Can you work these out from the model? Positions are in its coordinate system, mm. Round coordinates to 2 decimals unless told otherwise and drop trailing zeros. Loops run counter-clockwise (first coordinate to the right, second up) from the corner with the lowest first, then second, coordinate; pieces in that order, holes last. Notation, with made-up numbers: (18.25, 25) -> (75.25, 25) arc R25 ccw to (75.25, 41) -> close; hole circle Ø1 at (-34.5, 38). An arc over 180 degrees is marked (long way). Answer as a JSON object with one key per item and string values.
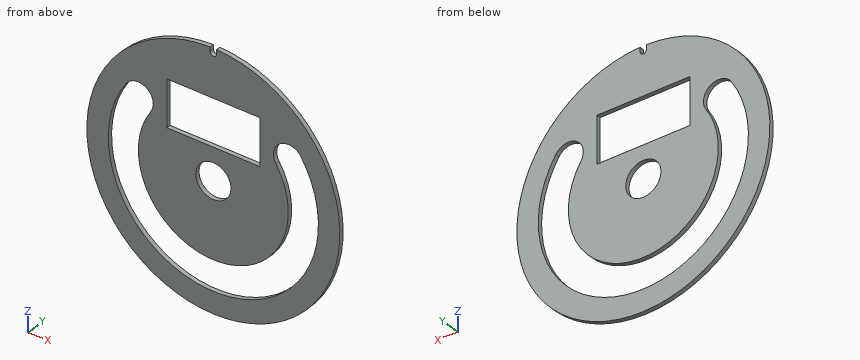
```python
from build123d import *

# Parameters (mm, degrees)
SKETCH_1_R      = 4.1
SKETCH_1_W      = 21.7
SKETCH_1_H      = 10.85
EXTRUDE_1_DEPTH = 1


with BuildPart() as part:
    # Эскиз1 → Бобышка-Вытянуть1 (new body)
    with BuildSketch(Plane(origin=(0, 0, 0), x_dir=(1, 0, 0), z_dir=(0, 1, 0))):
        with BuildLine():
            Line((0.75, -28.503654365), (0.75, -29.46545647))
            ThreePointArc((0.75, -29.46545647), (0, 29.475), (-0.75, -29.46545647))
            Line((-0.75, -29.46545647), (-0.75, -28.503654365))
            ThreePointArc((-0.75, -28.503654365), (0, -27.732186207), (0.75, -28.503654365))
        make_face()
        Circle(SKETCH_1_R, mode=Mode.SUBTRACT)
        with Locations((0, -12.957484911)):
            Rectangle(SKETCH_1_W, SKETCH_1_H, mode=Mode.SUBTRACT)
        with BuildLine():
            ThreePointArc((20.420143027, -13.492345376), (0, 24.475), (-20.420143027, -13.492345376))
            ThreePointArc((-20.420143027, -13.492345376), (-15.570553266, -14.483041669), (-14.579856973, -9.633451908))
            ThreePointArc((-14.579856973, -9.633451908), (0, 17.475), (14.579856973, -9.633451908))
            ThreePointArc((14.579856973, -9.633451908), (15.570553266, -14.483041669), (20.420143027, -13.492345376))
        make_face(mode=Mode.SUBTRACT)
    extrude(amount=EXTRUDE_1_DEPTH)


solid = part.part
```
Q1. I want a section at D-D, the plane y = 0.7. Write out the boundary of the cut face in (x, z) (3 decimals).
Determined:
{"outline": "(-0.75, 28.504) -> (-0.75, 29.465) arc R29.475 ccw (long way) to (0.75, 29.465) -> (0.75, 28.504) arc R0.75 cw (long way) to start; hole (-20.42, 13.492) arc R24.475 ccw (long way) to (20.42, 13.492) arc R3.5 ccw to (14.58, 9.633) arc R17.475 cw (long way) to (-14.58, 9.633) arc R3.5 ccw to start; hole (-10.85, 7.532) -> (10.85, 7.532) -> (10.85, 18.382) -> (-10.85, 18.382) -> close; hole circle Ø8.2 at (0, 0)"}
Q2. I'm going to push flat-ended pins straight in: pin 1 (0.5 mm diameter, centred on x = 4, y = 0.5, fed in from +Z); pin 2 (0.5 mm diameter, centred on x = 2, y = 0.5, fed in from -Z); pin 3 (4 mm diameter, centred on x = 16.5, z = 9, fed in from -Y). Where does each tip first touch, or does it pass through?
Determined:
{"pin 1": "z = 29.24", "pin 2": "z = -29.42", "pin 3": "y = 0"}
Q3. I want a section at C-C, the plane z = -8. Write out the boundary of the cut face in (x, y), then the cut area to 3 significant figures.
Determined:
{"outline": "(-28.37, 0) -> (-23.13, 0) -> (-23.13, 1) -> (-28.37, 1) -> close; (-15.54, 0) -> (15.54, 0) -> (15.54, 1) -> (-15.54, 1) -> close; (23.13, 0) -> (28.37, 0) -> (28.37, 1) -> (23.13, 1) -> close", "area": "41.5 mm²"}
Q4. I want a section at B-B, the plane z = 0. Write out the boundary of the cut face in (x, y) (3 decimals), then the cut area to 4 significant figures.
Determined:
{"outline": "(-29.475, 0) -> (-24.475, 0) -> (-24.475, 1) -> (-29.475, 1) -> close; (-17.475, 0) -> (-4.1, 0) -> (-4.1, 1) -> (-17.475, 1) -> close; (4.1, 0) -> (17.475, 0) -> (17.475, 1) -> (4.1, 1) -> close; (24.475, 0) -> (29.475, 0) -> (29.475, 1) -> (24.475, 1) -> close", "area": "36.75 mm²"}
Q5. I want a section at A-A, the plane x = 0. Write out the boundary of the cut face in (y, z) (3 decimals), then the cut area to 3 significant figures.
Determined:
{"outline": "(0, -29.475) -> (1, -29.475) -> (1, -24.475) -> (0, -24.475) -> close; (0, -17.475) -> (1, -17.475) -> (1, -4.1) -> (0, -4.1) -> close; (0, 4.1) -> (1, 4.1) -> (1, 7.532) -> (0, 7.532) -> close; (0, 18.382) -> (1, 18.382) -> (1, 27.732) -> (0, 27.732) -> close", "area": "31.2 mm²"}
Q6. If I drill on L1, parallel to X at y = 0.65, z = 0 (3 decimals); L2, parallel to Z at x = -6.5, y = 0.6; L3, parallel to Z at x = -14.5, y = 0.15, over which ranges is the centre line in solid material (lowest first)? Write a range as [from, to].
Determined:
{"L1": "[-29.475, -24.475], [-17.475, -4.1], [4.1, 17.475], [24.475, 29.475]", "L2": "[-28.75, -23.6], [-16.22, 7.53], [18.38, 28.75]", "L3": "[-25.66, -19.72], [-9.75, 9.76], [13.37, 25.66]"}
